Source: CAD feature listing. Evaluate the final solid. Frame: model axes, mm. A direction names the side the tool comes from. Give positions to 0.01 mm unless a question says otherwise; leave off trailing zeros. Loops run counter-clockwise (first coordinate to the right, second up) from the corner with the lowest first, then second, coordinate; pieces in that order, holes last. Notation, with made-up numbers: (58, 89) -> (107, 89) arc R19 ccw to (107, 109) -> close; hole circle Ø7 at (57, -17). An arc over 180 degrees is marked (long way). Put each result on its own line as item: value.
```python
from build123d import *

# Parameters (mm, degrees)
BOSS_EXTRUDE1_DEPTH = 10
SKETCH22_R          = 7.25
BOSS_EXTRUDE4_DEPTH = 10
SKETCH24_R          = 7.256494522
CUT_EXTRUDE15_DEPTH = 35
CUT_EXTRUDE16_DEPTH = 7
CIRPATTERN1_COUNT   = 4


with BuildPart() as part:
    # Sketch1 → Boss-Extrude1 (new body)
    with BuildSketch(Plane.XY):
        with BuildLine():
            Line((-5.05, 9.05), (5.05, 9.05))
            ThreePointArc((5.05, 9.05), (7.878427125, 7.878427125), (9.05, 5.05))
            Line((9.05, 5.05), (9.05, -5.05))
            ThreePointArc((9.05, -5.05), (7.878427125, -7.878427125), (5.05, -9.05))
            Line((5.05, -9.05), (-5.05, -9.05))
            ThreePointArc((-5.05, -9.05), (-7.878427125, -7.878427125), (-9.05, -5.05))
            Line((-9.05, -5.05), (-9.05, 5.05))
            ThreePointArc((-9.05, 5.05), (-7.878427125, 7.878427125), (-5.05, 9.05))
        make_face()
    extrude(amount=BOSS_EXTRUDE1_DEPTH)

    # Sketch22 → Boss-Extrude4 (add)
    with BuildSketch(Plane.XY.offset(10)):
        Polygon((-5.006494522, -7.75), (4.993505478, -7.75), (7.75, -5.003911735), (7.75, 4.996088265), (4.993505478, 7.75), (-5.006494522, 7.75), (-7.75, 4.996088265), (-7.75, -5.003911735), align=None)
        with Locations((-0.006494522, 0)):
            Circle(SKETCH22_R, mode=Mode.SUBTRACT)
    extrude(amount=BOSS_EXTRUDE4_DEPTH)

    # Sketch24 → Cut-Extrude15 (cut)
    with BuildSketch(Plane.XY.offset(10)):
        with Locations(Location((0, 0, 0), (0, 0, 180))):
            Circle(SKETCH24_R)
    extrude(amount=-CUT_EXTRUDE15_DEPTH, mode=Mode.SUBTRACT)

    # Sketch25 → Cut-Extrude16 (cut)
    with BuildSketch(Plane.XY.offset(20)):
        Polygon((0, 0), (7.75, 0.65), (7.75, -0.65), align=None)
    cut_extrude16 = extrude(amount=-CUT_EXTRUDE16_DEPTH, mode=Mode.SUBTRACT)

    # CirPattern1: Cut-Extrude16 ×4 about axis
    cirpattern1_axis = Axis((-0.006494522, 0, 20), (0, 0, -1))
    for i in range(1, CIRPATTERN1_COUNT):
        add(cut_extrude16.rotate(cirpattern1_axis, i * 360 / CIRPATTERN1_COUNT), mode=Mode.SUBTRACT)


solid = part.part
```
(1) Reachability of faces 1 (the flat face through (7.75, -1, 15)), 2 (the flat face through (1, 7.75, 15)), 3 (the flat face through (1, -7.75, 15)), 4 (the flat face through (6.391, 6.354, 14.93)) from +Z, -Z, +X, -X, +Y, -Y: full face, straight path, thin tool, end or side. Return the list, or none.
Calculated:
face 1: +Z, +X, +Y, -Y
face 2: +Z, +X, -X, +Y
face 3: +Z, +X, -X, -Y
face 4: +Z, +X, +Y
(2) Line query: probe 1 along Y at (x, z) = (0, 4.75); probe 2 along X at (y, z) = (-5.75, 14.25); probe 3 along Y at (x, z) = (-8, 4.75). Output: solid intervals per line, ascending. Write a range as from..to.
Calculated:
probe 1: y = -9.05..-7.26, 7.26..9.05
probe 2: x = -7..-4.42, 4.41..7
probe 3: y = -7.75..7.75
(3) Draft query along Y for faces 5 (the cylindrical face through (-7.847, -7.909, 4.93)), 6 (the flat face through (-9.05, 0, 5)), 7 (the cylindrical face through (7.847, 7.909, 4.93)), 8 (the cylindrical face through (6.69, -2.78, 14.93)). Return one class per face: released by +Y, released by -Y, zero draft, split by the parting line, or undercut.
Calculated:
face 5: released by -Y
face 6: zero draft
face 7: released by +Y
face 8: undercut
(4) Section D-D on z = 17.75. Return loops of the section in (x, y), then the cut area to 3 significant figures.
Calculated:
outline: (-7.75, -5) -> (-5.01, -7.75) -> (-0.66, -7.75) -> (-0.61, -7.22) arc R7.25 cw to (-7.23, -0.61) -> (-7.75, -0.65) -> close; (-7.75, 0.65) -> (-7.23, 0.61) arc R7.25 cw to (-0.61, 7.22) -> (-0.66, 7.75) -> (-5.01, 7.75) -> (-7.75, 5) -> close; (0.6, -7.22) -> (0.64, -7.75) -> (4.99, -7.75) -> (7.75, -5) -> (7.75, -0.65) -> (7.22, -0.61) arc R7.25 cw to start; (0.6, 7.22) arc R7.25 cw to (7.22, 0.61) -> (7.75, 0.65) -> (7.75, 5) -> (4.99, 7.75) -> (0.64, 7.75) -> close
area: 57.4 mm²
(5) First-contact query: P1, Ø5, axis at x = 1.5, y = -5, coming from the +Z side; P2, Ø8, axis at y = 2, z = 16.5, coming from the -X side; P3, Ø1.5, axis at y = 7, z = 6, coming from the -X side; P4, Ø1, axis at x = 5, z = 11, coming from the -Y side. Flat tips, straight axial feed; report the tip coordinate or a pass-through.
Calculated:
P1: stops at z = 20
P2: stops at x = -7.75
P3: stops at x = -8.87
P4: stops at y = -7.75
(6) Section B-B on z = 12. Return loops of the section in (x, y).
Calculated:
outline: (-7.75, -5) -> (-5.01, -7.75) -> (4.99, -7.75) -> (7.75, -5) -> (7.75, 5) -> (4.99, 7.75) -> (-5.01, 7.75) -> (-7.75, 5) -> close; hole circle Ø14.5 at (-0.01, 0)
